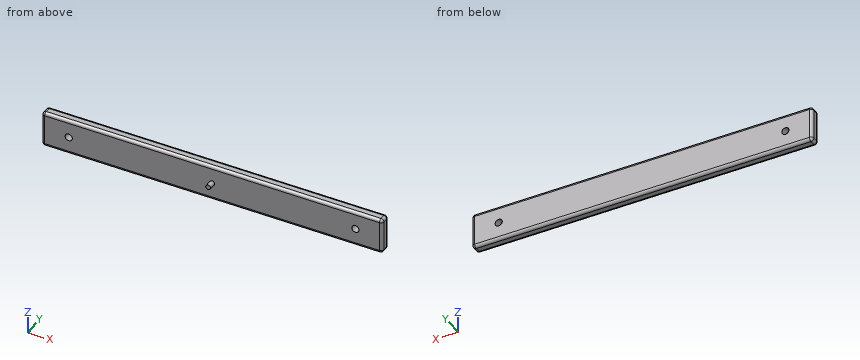
```python
from build123d import *

# Parameters (mm, degrees)
SKETCH1_W           = 95
SKETCH1_H           = 10
BOSS_EXTRUDE1_DEPTH = 3
FILLET1_R           = 0.8
FILLET2_R           = 0.8
SKETCH2_R           = 1
CUT_EXTRUDE1_DEPTH  = 48.8565565
SKETCH3_R           = 1
BOSS_EXTRUDE2_DEPTH = 5
CUT_EXTRUDE3_START  = -2
SKETCH4_R           = 1
SKETCH4_R_2         = 0.678596162
CUT_EXTRUDE3_DEPTH  = 2


with BuildPart() as part:
    # Sketch1 → Boss-Extrude1 (new body)
    with BuildSketch(Plane(origin=(0, 0, 0), x_dir=(1, 0, 0), z_dir=(0, 1, 0))):
        Rectangle(SKETCH1_W, SKETCH1_H)
    extrude(amount=BOSS_EXTRUDE1_DEPTH)

    # Fillet1
    fillet1_edges = [part.edges().sort_by_distance(p)[0] for p in [
        (-47.5, 3, 0),
        (0, 3, 5),
        (47.5, 3, 0),
        (0, 0, 5),
        (-47.5, 0, 0),
        (0, 0, -5),
        (47.5, 0, 0),
        (0, 3, -5),
    ]]
    fillet(fillet1_edges, radius=FILLET1_R)

    # Fillet2
    # the kernel refuses this fillet: 0.8 mm, written as the material it takes off along each edge
    with BuildSketch(Plane(origin=(46.7, 0.8, 4.2), x_dir=(0, 0, 1), z_dir=(1, 0, 0))) as fillet2_piece_1_section:
        Polygon((0, 0), (FILLET2_R, 0), (FILLET2_R, FILLET2_R), (0, FILLET2_R), align=None)
    fillet2_piece_1 = extrude(amount=FILLET2_R, mode=Mode.PRIVATE)
    fillet2_piece_1 = fillet2_piece_1 - Plane(origin=(46.7, 0.8, 4.2), x_dir=(0, 0.7071067811865475, -0.7071067811865475), z_dir=(1, 0, 0)) * Sphere(FILLET2_R, mode=Mode.PRIVATE)
    add(fillet2_piece_1, mode=Mode.SUBTRACT)
    with BuildSketch(Plane(origin=(-46.7, 0.8, 4.2), x_dir=(0, 0, 1), z_dir=(-1, 0, 0))) as fillet2_piece_2_section:
        Polygon((0, 0), (FILLET2_R, 0), (FILLET2_R, -FILLET2_R), (0, -FILLET2_R), align=None)
    fillet2_piece_2 = extrude(amount=FILLET2_R, mode=Mode.PRIVATE)
    fillet2_piece_2 = fillet2_piece_2 - Plane(origin=(-46.7, 0.8, 4.2), x_dir=(0, 0.7071067811865475, -0.7071067811865475), z_dir=(-1, 0, 0)) * Sphere(FILLET2_R, mode=Mode.PRIVATE)
    add(fillet2_piece_2, mode=Mode.SUBTRACT)
    with BuildSketch(Plane(origin=(46.7, 0.8, -4.2), x_dir=(1, 0, 0), z_dir=(0, 0, -1))) as fillet2_piece_3_section:
        Polygon((0, 0), (FILLET2_R, 0), (FILLET2_R, FILLET2_R), (0, FILLET2_R), align=None)
    fillet2_piece_3 = extrude(amount=FILLET2_R, mode=Mode.PRIVATE)
    fillet2_piece_3 = fillet2_piece_3 - Plane(origin=(46.7, 0.8, -4.2), x_dir=(-0.7071067811865475, 0.7071067811865475, 0), z_dir=(0, 0, -1)) * Sphere(FILLET2_R, mode=Mode.PRIVATE)
    add(fillet2_piece_3, mode=Mode.SUBTRACT)
    with BuildSketch(Plane(origin=(-46.7, 0.8, -4.2), x_dir=(-1, 0, 0), z_dir=(0, 0, -1))) as fillet2_piece_4_section:
        Polygon((0, 0), (FILLET2_R, 0), (FILLET2_R, -FILLET2_R), (0, -FILLET2_R), align=None)
    fillet2_piece_4 = extrude(amount=FILLET2_R, mode=Mode.PRIVATE)
    fillet2_piece_4 = fillet2_piece_4 - Plane(origin=(-46.7, 0.8, -4.2), x_dir=(0.7071067811865475, 0.7071067811865475, 0), z_dir=(0, 0, -1)) * Sphere(FILLET2_R, mode=Mode.PRIVATE)
    add(fillet2_piece_4, mode=Mode.SUBTRACT)
    with BuildSketch(Plane(origin=(-46.7, 2.2, -4.2), x_dir=(-1, 0, 0), z_dir=(0, 0, -1))) as fillet2_piece_5_section:
        Polygon((0, 0), (FILLET2_R, 0), (FILLET2_R, FILLET2_R), (0, FILLET2_R), align=None)
    fillet2_piece_5 = extrude(amount=FILLET2_R, mode=Mode.PRIVATE)
    fillet2_piece_5 = fillet2_piece_5 - Plane(origin=(-46.7, 2.2, -4.2), x_dir=(0.7071067811865475, -0.7071067811865475, 0), z_dir=(0, 0, -1)) * Sphere(FILLET2_R, mode=Mode.PRIVATE)
    add(fillet2_piece_5, mode=Mode.SUBTRACT)
    with BuildSketch(Plane(origin=(46.7, 2.2, -4.2), x_dir=(1, 0, 0), z_dir=(0, 0, -1))) as fillet2_piece_6_section:
        Polygon((0, 0), (FILLET2_R, 0), (FILLET2_R, -FILLET2_R), (0, -FILLET2_R), align=None)
    fillet2_piece_6 = extrude(amount=FILLET2_R, mode=Mode.PRIVATE)
    fillet2_piece_6 = fillet2_piece_6 - Plane(origin=(46.7, 2.2, -4.2), x_dir=(-0.7071067811865475, -0.7071067811865475, 0), z_dir=(0, 0, -1)) * Sphere(FILLET2_R, mode=Mode.PRIVATE)
    add(fillet2_piece_6, mode=Mode.SUBTRACT)
    with BuildSketch(Plane(origin=(-46.7, 2.2, 4.2), x_dir=(0, 0, 1), z_dir=(-1, 0, 0))) as fillet2_piece_7_section:
        Polygon((0, 0), (FILLET2_R, 0), (FILLET2_R, FILLET2_R), (0, FILLET2_R), align=None)
    fillet2_piece_7 = extrude(amount=FILLET2_R, mode=Mode.PRIVATE)
    fillet2_piece_7 = fillet2_piece_7 - Plane(origin=(-46.7, 2.2, 4.2), x_dir=(0, -0.7071067811865475, -0.7071067811865475), z_dir=(-1, 0, 0)) * Sphere(FILLET2_R, mode=Mode.PRIVATE)
    add(fillet2_piece_7, mode=Mode.SUBTRACT)
    with BuildSketch(Plane(origin=(46.7, 2.2, 4.2), x_dir=(0, 0, 1), z_dir=(1, 0, 0))) as fillet2_piece_8_section:
        Polygon((0, 0), (FILLET2_R, 0), (FILLET2_R, -FILLET2_R), (0, -FILLET2_R), align=None)
    fillet2_piece_8 = extrude(amount=FILLET2_R, mode=Mode.PRIVATE)
    fillet2_piece_8 = fillet2_piece_8 - Plane(origin=(46.7, 2.2, 4.2), x_dir=(0, -0.7071067811865475, -0.7071067811865475), z_dir=(1, 0, 0)) * Sphere(FILLET2_R, mode=Mode.PRIVATE)
    add(fillet2_piece_8, mode=Mode.SUBTRACT)
    with BuildSketch(Plane(origin=(-47.5, 0.8, -5), x_dir=(1, 0, 0), z_dir=(0, 1, 0)), Plane(origin=(-47.5, 0.8, 5), x_dir=(0, 0, -1), z_dir=(0, 1, 0))) as fillet2_piece_9:
        with BuildLine():
            CenterArc((FILLET2_R, -FILLET2_R), FILLET2_R, 90, 90)
            Line((0, -FILLET2_R), (0, 0))
            Line((0, 0), (FILLET2_R, 0))
        make_face()
    extrude(amount=1.4, mode=Mode.SUBTRACT)
    with BuildSketch(Plane(origin=(47.5, 0.8, -5), x_dir=(-1, 0, 0), z_dir=(0, 1, 0)), Plane(origin=(47.5, 0.8, 5), x_dir=(0, 0, -1), z_dir=(0, 1, 0))) as fillet2_piece_10:
        with BuildLine():
            CenterArc((FILLET2_R, FILLET2_R), FILLET2_R, 180, 90)
            Line((0, FILLET2_R), (0, 0))
            Line((0, 0), (FILLET2_R, 0))
        make_face()
    extrude(amount=1.4, mode=Mode.SUBTRACT)

    # Sketch2 → Cut-Extrude1 (cut, through all)
    with BuildSketch(Plane(origin=(0, 3, 0), x_dir=(1, 0, 0), z_dir=(0, 1, 0))):
        with Locations(Location((0, 0, 0), (0, 0, 270))):
            Circle(SKETCH2_R)
        with Locations(Location((-40, 0, 0), (0, 0, 270))):
            Circle(SKETCH2_R)
        with Locations(Location((40, 0, 0), (0, 0, 270))):
            Circle(SKETCH2_R)
    extrude(amount=-CUT_EXTRUDE1_DEPTH, mode=Mode.SUBTRACT)

    # Sketch3 → Boss-Extrude2 (add)
    with BuildSketch(Plane(origin=(0, 3, 0), x_dir=(1, 0, 0), z_dir=(0, 1, 0))):
        with Locations(Location((0, 0, 0), (0, 0, 270))):
            Circle(SKETCH3_R)
    extrude(amount=-BOSS_EXTRUDE2_DEPTH)

    # Sketch4 → Cut-Extrude3 (cut)
    with BuildSketch(Plane.XZ.offset(2).offset(CUT_EXTRUDE3_START)):
        Circle(SKETCH4_R)
        with Locations(Location((0, 0, 0), (0, 0, 270))):
            Circle(SKETCH4_R_2, mode=Mode.SUBTRACT)
    extrude(amount=CUT_EXTRUDE3_DEPTH, mode=Mode.SUBTRACT)


solid = part.part
```
Geometry: final body of the model. Coordinates: model frame, mm. Coordinates: 2 decimals unless noted, no trailing zeros. Order: outer loops, then holes, each group sorted by start corner. A loop starts at its lowest first (then second) coordinate and runs counter-clockwise, first axis right, second up. Notation, with made-up numbers: (64, 15) - (119, 15) arc R35 ccw to (119, 52) - close; hole circle Ø3 at (-34, 46). An arc over 180 degrees is marked (long way). Return JSON: item names as keys, results as strings. Group by question number.
1. Cut plane B-B (x = -19). Output: boundary loops of the cut face in (y, z), plus the area to 3 significant figures.
2. Material intervals for line 1 along X through (y, z) = (2, 0); line 2 along Y through (x, z) = (-4, -0.25); line 3 along Y through (x, z) = (35.5, 4.75), sorted ascending. Write a range as [from, to].
3. Cut plane D-D (y = -1.05). Output: boundary loops of the cut face in (x, z), plus the area to 3 significant figures.
4. Cut plane C-C (z = -3). Output: boundary loops of the cut face in (x, y).
5. Cut plane A-A (x = 40). Output: boundary loops of the cut face in (y, z), plus the area to 3 significant figures.
6. Pin query (flat end, axial travel): pin 1 (1 mm diameter, centred on x = -31.5, z = -2.5, fed in from -Y); pin 2 (1 mm diameter, centred on x = -35.5, y = 0, fed in from -Z). Return the tip coordinate at first contact, or that it passes through.
Resolved:
{
 "1": {"outline": "(0, -4.2) arc R0.8 ccw to (0.8, -5) - (2.2, -5) arc R0.8 ccw to (3, -4.2) - (3, 4.2) arc R0.8 ccw to (2.2, 5) - (0.8, 5) arc R0.8 ccw to (0, 4.2) - close", "area": "29.5 mm²"},
 "2": {"line 1": "x = [-47.5, -41], [-39, 39], [41, 47.5]", "line 2": "y = [0, 3]", "line 3": "y = [0.22, 2.78]"},
 "3": {"outline": "circle Ø1.36 at (0, 0)", "area": "1.45 mm²"},
 "4": {"outline": "(-47.5, 0.8) arc R0.8 ccw to (-46.7, 0) - (46.7, 0) arc R0.8 ccw to (47.5, 0.8) - (47.5, 2.2) arc R0.8 ccw to (46.7, 3) - (-46.7, 3) arc R0.8 ccw to (-47.5, 2.2) - close"},
 "5": {"outline": "(0, -4.2) arc R0.8 ccw to (0.8, -5) - (2.2, -5) arc R0.8 ccw to (3, -4.2) - (3, -1) - (0, -1) - close; (0, 1) - (3, 1) - (3, 4.2) arc R0.8 ccw to (2.2, 5) - (0.8, 5) arc R0.8 ccw to (0, 4.2) - close", "area": "23.5 mm²"},
 "6": {"pin 1": "stops at y = 0", "pin 2": "stops at z = -4.94"}
}
